Build history of the part. All positions in model axes, mm. Face numbers are marked on the shaded views. Round coordinates to 2 decimals unless told otherwise and drop trailing zeros. Write each loop counter-clockwise with the first axis right and the second up, starting at its lowest first coordinate (ties: lowest second). Pieces come first, ordered by that corner, then holes. Notation, with made-up numbers: (81, 18.5) -> (119, 18.5) arc R17 cw to (119, 22.5) -> close; hole circle Ø6 at (-2.75, 21.25). An arc over 180 degrees is marked (long way). One line per question, with ' | ' between items.
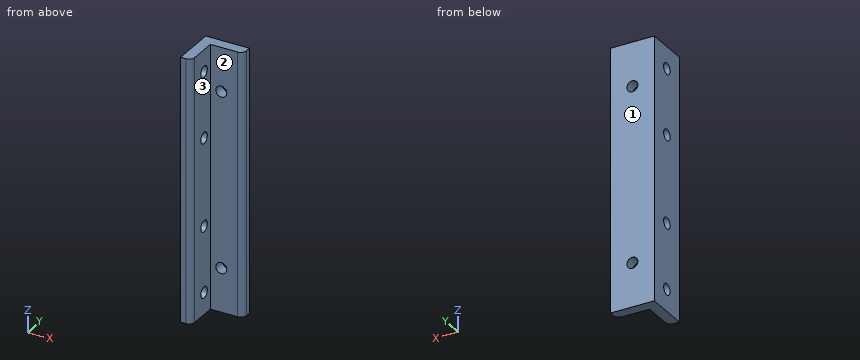
from build123d import *

# Parameters (mm, degrees)
F1_DEPTH = 152.4
F4_D     = 6.35
F4_DEPTH = 25.4
F5_D     = 6.5278
F5_DEPTH = 25.4


with BuildPart() as f1:
    # F0 (on Top) → F1 (new body)
    with BuildSketch(Plane.XY):
        with BuildLine():
            Line((25.4, 0), (0, 0))
            Line((0, 0), (0, -25.4))
            Line((0, -25.4), (3.175, -25.4))
            ThreePointArc((3.175, -25.4), (5.420064, -24.470064), (6.35, -22.225))
            Line((6.35, -22.225), (6.35, -19.05))
            Line((6.35, -19.05), (6.35, -6.35))
            Line((6.35, -6.35), (18.926421, -6.35))
            Line((18.926421, -6.35), (19.173579, -6.35))
            Line((19.173579, -6.35), (22.225, -6.35))
            ThreePointArc((22.225, -6.35), (24.470064, -5.420064), (25.4, -3.175))
            Line((25.4, -3.175), (25.4, -0.001203))
            Line((25.4, -0.001203), (25.4, 0))
        make_face()
    extrude(amount=F1_DEPTH)

    # F4
    with Locations(Plane(origin=(0, 0, 0), x_dir=(-1, 0, 0), z_dir=(0, 1, 0))):
        with Locations((-12.7, 127), (-12.7, 25.4)):
            Hole(F4_D / 2, depth=F4_DEPTH)

    # F5
    with Locations(Plane(origin=(0, 0, 0), x_dir=(0, -1, 0), z_dir=(-1, 0, 0))):
        with Locations((12.7, 12.7), (12.7, 50.8), (12.7, 101.6), (12.7, 139.7)):
            Hole(F5_D / 2, depth=F5_DEPTH)


solid = f1.part
(1) Slice it at D-D (y = -1.5). Write the cut outline in (x, z) (3 decimals).
Calculated:
outline: (0, 0) -> (25.4, 0) -> (25.4, 152.4) -> (0, 152.4) -> close; hole circle Ø6.35 at (12.7, 25.4); hole circle Ø6.35 at (12.7, 127)
(2) Slice it at A-A (z = 127). Write the cut outline in (x, y) (3 decimals), then the cut area to 3 significant figures.
Calculated:
outline: (0, -25.4) -> (3.175, -25.4) arc R3.175 ccw to (6.35, -22.225) -> (6.35, -6.35) -> (9.525, -6.35) -> (9.525, 0) -> (0, 0) -> close; (15.875, -6.35) -> (22.225, -6.35) arc R3.175 ccw to (25.4, -3.175) -> (25.4, 0) -> (15.875, 0) -> close | area: 238 mm2
(3) Wall check: line 1 (Z direction, x = 12.7, y = -3) (3 decimals); line 2 (Z direction, x = 2.25, y = -13); line 3 (Z direction, x = 2.75, y = -12.7). Give the ranges that are in metal, low to high. Write a range as from..to.
Calculated:
line 1: 0..22.225, 28.575..123.825, 130.175..152.4 | line 2: 0..9.45, 15.95..47.55, 54.05..98.35, 104.85..136.45, 142.95..152.4 | line 3: 0..9.44, 15.96..47.54, 54.06..98.34, 104.86..136.44, 142.96..152.4
(4) Drop flat-ended pins along their axis: pin 1 (7.5 mm diameter, centred on y = -12.7, z = 50.8, fed in from -X); pin 2 (5 mm diameter, centred on y = -12.7, z = 139.7, fed in from +X); pin 3 (8.5 mm diameter, centred on y = -12.7, z = 12.7, fed in from +X); pin 4 (1 mm diameter, centred on x = 20.5, z = 35.5, fed in from -Y). Give the stop position or say it passes through.
Calculated:
pin 1: x = 0 | pin 2: through | pin 3: x = 6.35 | pin 4: y = -6.35
(5) Slice it at B-B (x = 12.7). Write the cut outline in (y, z) (3 decimals).
Calculated:
outline: (-6.35, 0) -> (0, 0) -> (0, 22.225) -> (-6.35, 22.225) -> close; (-6.35, 28.575) -> (0, 28.575) -> (0, 123.825) -> (-6.35, 123.825) -> close; (-6.35, 130.175) -> (0, 130.175) -> (0, 152.4) -> (-6.35, 152.4) -> close
(6) Mould opens along Y. For the marked faces 1, 2 and 3 say: pulls with the +Y half, pulls with the -Y half, needs draft (parallel to the pull), parting line crosses it, or undercut.
Calculated:
face 1: pulls with the +Y half | face 2: pulls with the -Y half | face 3: needs draft
(7) Slice it at C-C (y = -12). Write the cut outline in (x, z).
Calculated:
outline: (0, 0) -> (6.35, 0) -> (6.35, 9.51) -> (0, 9.51) -> close; (0, 15.89) -> (6.35, 15.89) -> (6.35, 47.61) -> (0, 47.61) -> close; (0, 53.99) -> (6.35, 53.99) -> (6.35, 98.41) -> (0, 98.41) -> close; (0, 104.79) -> (6.35, 104.79) -> (6.35, 136.51) -> (0, 136.51) -> close; (0, 142.89) -> (6.35, 142.89) -> (6.35, 152.4) -> (0, 152.4) -> close
